from build123d import *

# Parameters (mm, degrees)
SKETCH_1_R      = 2.5
SKETCH_1_R_2    = 2
SKETCH_1_R_3    = 1.5
EXTRUDE_1_DEPTH = 3
FILLET_1_R      = 20
FILLET_2_R      = 5


with BuildPart() as part:
    # 草图1 → 凸台-拉伸1 (new body)
    with BuildSketch(Plane(origin=(0, 0, 0), x_dir=(1, 0, 0), z_dir=(0, 1, 0))):
        with BuildLine():
            Line((-72.5, -61.5), (-40, -61.5))
            Line((-40, -61.5), (-34.965402213, -67.5))
            Line((-34.965402213, -67.5), (34.965402213, -67.5))
            Line((34.965402213, -67.5), (40, -61.5))
            Line((40, -61.5), (72.5, -61.5))
            Line((72.5, -61.5), (72.5, -35.669872981))
            ThreePointArc((72.5, -35.669872981), (73.011112606, -31.787587305), (74.509618943, -28.169872981))
            Line((74.509618943, -28.169872981), (89.330127019, -2.5))
            ThreePointArc((89.330127019, -2.5), (88.512514494, 3.558404408), (82.444008336, 4.297313883))
            Line((82.444008336, 4.297313883), (50, -15))
            Line((50, -15), (35, -15))
            Line((35, -15), (35, -45))
            ThreePointArc((35, -45), (34.121320344, -47.121320344), (32, -48))
            Line((32, -48), (-32, -48))
            ThreePointArc((-32, -48), (-34.121320344, -47.121320344), (-35, -45))
            Line((-35, -45), (-35, -15))
            Line((-35, -15), (-50, -15))
            Line((-50, -15), (-82.444008336, 4.297313883))
            ThreePointArc((-82.444008336, 4.297313883), (-88.512514494, 3.558404408), (-89.330127019, -2.5))
            Line((-89.330127019, -2.5), (-74.509618943, -28.169872981))
            ThreePointArc((-74.509618943, -28.169872981), (-73.011112606, -31.787587305), (-72.5, -35.669872981))
            Line((-72.5, -35.669872981), (-72.5, -61.5))
        make_face()
        with Locations(Location((85, 0, 0), (0, 0, 270))):
            Circle(SKETCH_1_R, mode=Mode.SUBTRACT)
        with Locations(Location((-85, 0, 0), (0, 0, 270))):
            Circle(SKETCH_1_R, mode=Mode.SUBTRACT)
        with Locations(Location((47.5, -27, 0), (0, 0, 270))):
            Circle(SKETCH_1_R_2, mode=Mode.SUBTRACT)
        with Locations(Location((47.5, -52, 0), (0, 0, 270))):
            Circle(SKETCH_1_R_2, mode=Mode.SUBTRACT)
        with Locations(Location((-47.5, -52, 0), (0, 0, 270))):
            Circle(SKETCH_1_R_2, mode=Mode.SUBTRACT)
        with Locations(Location((-47.5, -27, 0), (0, 0, 270))):
            Circle(SKETCH_1_R_2, mode=Mode.SUBTRACT)
        with Locations(Location((-20, -55.5, 0), (0, 0, 270))):
            Circle(SKETCH_1_R_3, mode=Mode.SUBTRACT)
        with Locations(Location((20, -55.5, 0), (0, 0, 270))):
            Circle(SKETCH_1_R_3, mode=Mode.SUBTRACT)
        with Locations(Location((65, -55.5, 0), (0, 0, 270))):
            Circle(SKETCH_1_R_3, mode=Mode.SUBTRACT)
        with Locations(Location((-65, -55.5, 0), (0, 0, 270))):
            Circle(SKETCH_1_R_3, mode=Mode.SUBTRACT)
        with Locations(Location((65, -20, 0), (0, 0, 270))):
            Circle(SKETCH_1_R_3, mode=Mode.SUBTRACT)
        with Locations(Location((-65, -20, 0), (0, 0, 270))):
            Circle(SKETCH_1_R_3, mode=Mode.SUBTRACT)
    extrude(amount=EXTRUDE_1_DEPTH)

    # 圆角1
    fillet_1_edges = [part.edges().sort_by_distance(p)[0] for p in [
        (50, 1.5, 15),
        (-50, 1.5, 15),
    ]]
    fillet(fillet_1_edges, radius=FILLET_1_R)

    # 圆角2
    fillet_2_edges = [part.edges().sort_by_distance(p)[0] for p in [
        (-35, 1.5, 15),
        (35, 1.5, 15),
        (72.5, 1.5, 61.5),
        (40, 1.5, 61.5),
        (34.965402213, 1.5, 67.5),
        (-34.965402213, 1.5, 67.5),
        (-40, 1.5, 61.5),
        (-72.5, 1.5, 61.5),
    ]]
    fillet(fillet_2_edges, radius=FILLET_2_R)


solid = part.part
Could you check a few things on this model? Use its own coordinates, in mm. A direction names the side the tool comes from. Give positions to 0.01 mm unless a question says otherwise; leave off trailing zeros. Order: outer loops, then holes, each group sorted by start corner. A loop starts at its lowest first (then second) coordinate and runs counter-clockwise, first axis right, second up.
1. Will these pins go through, and if not, where does the flat tip stop? P1, Ø3, axis at x = -85, z = 0, coming from the -Y side; P2, Ø1.5, axis at x = -8, y = 1.5, coming from the -Z side; P3, Ø0.9, axis at y = 1.5, z = 50.5, coming from the +X side; P4, Ø0.9, axis at y = 1, z = 30, coming from the -X side.
2. I need wall thicknesses on L1, parallel to X at y = 0.6, z = 55.5; L2, parallel to X at y = 1.5, z = 52; L3, parallel to X at y = 2.7, z = -1.5. Which ranges of each line are inside material? Lowest first, please.
3. Suppose I cut it at D-D (z = 0). List the corners of the cut face in (x, y) for me, plus the area to 3 significant figures.
4. We'd pull the mould along X, two halves only. Please class faces 1 (the flat face through (81.82, 1.48, 15.51)), 2 (the cylindrical face through (-63.513, 1.479, 19.805)), 3 (the cylindrical face through (-73.025, 1.479, 31.735)): pulls with the +X half, pulls with the -X half, needs draft (parallel to the pull), parting line crosses it, or undercut.
5. Suppose I cut it at C-C (x = -47.5). List the corners of the cut face in (y, z) for me, plus the area to 3 significant figures.
6. Suppose I cut it at B-B (z = 37.5). List the corners of the cut face in (x, y) for me, plus the area to 3 significant figures.
7. Suppose I cut it at A-A (x = 85). List the corners of the cut face in (y, z) for me, plus the area to 3 significant figures.
8. For faces 4 (the cylindrical face through (-49.274, 1.479, 27.923)), 5 (the flat face through (-68.39, 1.48, 4.06)), 6 (the flat face through (55, 1, 61.5)), which set-ups out of +Z, -Z, +X, -X, +Y, -Y let a thin tool reach every point of the face, with its end or its side?
Solved:
1. P1: passes through
1. P2: stops at z = 48
1. P3: stops at x = 72.5
1. P4: stops at x = -73.81
2. L1: x = -72.5 to -66.5, -63.5 to -21.5, -18.5 to 18.5, 21.5 to 63.5, 66.5 to 72.5
2. L2: x = -72.5 to -49.5, -45.5 to 45.5, 49.5 to 72.5
2. L3: x = -89.77 to -87, -83 to -77.74, 77.74 to 83, 87 to 89.77
3. outline: (-90, 0) - (-87.5, 0) - (-87.5, 3) - (-90, 3) - close; (-82.5, 0) - (-75.22, 0) - (-75.22, 3) - (-82.5, 3) - close; (75.22, 0) - (82.5, 0) - (82.5, 3) - (75.22, 3) - close; (87.5, 0) - (90, 0) - (90, 3) - (87.5, 3) - close
3. area: 58.7 mm2
4. face 1: pulls with the +X half
4. face 2: undercut
4. face 3: pulls with the -X half
5. outline: (0, 14.77) - (3, 14.77) - (3, 25) - (0, 25) - close; (0, 29) - (3, 29) - (3, 50) - (0, 50) - close; (0, 54) - (3, 54) - (3, 61.5) - (0, 61.5) - close
5. area: 116 mm2
6. outline: (-72.5, 0) - (-35, 0) - (-35, 3) - (-72.5, 3) - close; (35, 0) - (72.5, 0) - (72.5, 3) - (35, 3) - close
6. area: 225 mm2
7. outline: (0, -5) - (3, -5) - (3, -2.5) - (0, -2.5) - close; (0, 2.5) - (3, 2.5) - (3, 10) - (0, 10) - close
7. area: 30.0 mm2
8. face 4: +Y, -Y
8. face 5: -Z, +Y, -Y
8. face 6: +Z, +X, +Y, -Y
